Here's how the part is built. I have some questions about the finished solid (model axes, mm). Face numbers are marked on the shaded views. A direction names the side the tool comes from. Coordinates: 2 decimals unless noted, no trailing zeros. Write each loop counter-clockwise with the first axis right and the second up, starting at its lowest first coordinate (ties: lowest second). Pieces come first, ordered by that corner, then holes.
Item 1: I want a section at A-A (z = 7). Please give me the cut outline in (x, y), and give its area (3 significant figures).
Item 2: I'm going to push flat-ended pins straight in: P1, Ø12, axis at y = -29, z = 18.5, coming from the +X side; P2, Ø3, axis at x = -17, y = -10, coming from the +Z side; P3, Ø3, axis at x = 28, z = 13, coming from the +Y side; P4, Ø5, axis at x = -1.5, y = -7, coming from the -Z side. Where does each tip first touch, or does it pass through?
Item 3: I want a section at C-C (y = 18.5). Please give me the cut outline in (x, z).
Item 4: For the marked faces 5, 6, 7, 8 and 9, which set-ups out of +Z, -Z, +X, -X, +Y, -Y let a thin tool reach every point of the face, with its end or its side?
Item 5: I want a section at B-B (x = -13.5). Please give me the cut outline in (y, z).
Item 6: Please list where these lines run through material, in increasing order: line 1 (X direction, y = 6, z = 30.5); line 2 (X direction, y = 35.5, z = 6); line 3 (Y direction, x = -12.5, z = 32).
Item 7: I want a section at D-D (x = 24). Please give me the cut outline in (y, z), and give its area (3 significant figures).
Item 8: If we mould it in two halves opening along Y, with no side actions, what happens to the marked faces 1, 2, 3 and 4? For each: pulls with the +Y half, pulls with the -Y half, needs draft (parallel to the pull), parting line crosses it, or undercut.
from build123d import *

# Parameters (mm, degrees)
EXTRUDE_1_DEPTH     = 34
SKETCH_4_R          = 3.85
SKETCH_4_R_2        = 2.85
EXTRUDE_2_DEPTH     = 16.5
SKETCH_5_R          = 1.85
CUT_EXTRUDE_2_DEPTH = 35
SKETCH_6_R          = 3
CUT_EXTRUDE_3_DEPTH = 4
SKETCH_7_W          = 34
SKETCH_7_H          = 5
EXTRUDE_3_DEPTH     = 15
FILLET_2_R          = 2.5
FILLET_3_R          = 2.5
FILLET_4_R          = 2.5
SKETCH_8_W          = 5
SKETCH_8_H          = 34
EXTRUDE_4_DEPTH     = 15
SKETCH_9_W          = 5
SKETCH_9_H          = 34
EXTRUDE_5_DEPTH     = 15
FILLET_5_R          = 2.5


with BuildPart() as part:
    # 草圖1 → 填料-伸長1 (new body)
    with BuildSketch(Plane.XY):
        Polygon((0.59122025, -5.441901053), (39.56236342, -27.941901053), (36.06236342, -34.00407888), (-2.90877975, -11.50407888), (-41.87992292, -34.00407888), (-45.37992292, -27.941901053), (-6.40877975, -5.441901053), (-6.40877975, 39.558098947), (0.59122025, 39.558098947), align=None)
    extrude(amount=EXTRUDE_1_DEPTH)

    # 草圖4 → 填料-伸長2 (add)
    with BuildSketch(Plane.XY.offset(34)):
        with Locations((-2.90877975, -7.462626996)):
            Circle(SKETCH_4_R)
        with Locations((-2.90877975, -7.462626996)):
            Circle(SKETCH_4_R_2, mode=Mode.SUBTRACT)
    extrude(amount=EXTRUDE_2_DEPTH)

    # 草圖5 → 除料-伸長2 (cut, through all)
    with BuildSketch(Plane.XY.offset(34)):
        with Locations((-2.90877975, -7.462626996)):
            Circle(SKETCH_5_R)
    extrude(amount=-CUT_EXTRUDE_2_DEPTH, mode=Mode.SUBTRACT)

    # 草圖6 → 除料-伸長3 (cut)
    with BuildSketch(Plane(origin=(0, 0, 0), x_dir=(-1, 0, 0), z_dir=(0, 0, -1))):
        with Locations((2.90877975, -7.462626996)):
            Circle(SKETCH_6_R)
    extrude(amount=-CUT_EXTRUDE_3_DEPTH, mode=Mode.SUBTRACT)

    # 草圖7 → 填料-伸長3 (add)
    with BuildSketch(Plane.ZY.offset(6.40877975)):
        with Locations((17, 37.058098947)):
            Rectangle(SKETCH_7_W, SKETCH_7_H)
    extrude(amount=EXTRUDE_3_DEPTH)

    # 圓角2
    fillet_2_edges = [part.edges().sort_by_distance(p)[0] for p in [
        (-21.40877975, 39.558098947, 17),
    ]]
    fillet(fillet_2_edges, radius=FILLET_2_R)

    # 圓角3
    fillet_3_edges = [part.edges().sort_by_distance(p)[0] for p in [
        (0.59122025, 39.558098947, 17),
    ]]
    fillet(fillet_3_edges, radius=FILLET_3_R)

    # 圓角4
    fillet_4_edges = [part.edges().sort_by_distance(p)[0] for p in [
        (-6.40877975, 34.558098947, 17),
    ]]
    fillet(fillet_4_edges, radius=FILLET_4_R)

    # 草圖8 → 填料-伸長4 (add)
    with BuildSketch(Plane(origin=(4.254217341, -7.368520581, 0), x_dir=(0.866025404, 0.5, 0), z_dir=(0.5, -0.866025404, 0))):
        with Locations((-50.771116598, 17)):
            Rectangle(SKETCH_8_W, SKETCH_8_H)
    extrude(amount=EXTRUDE_4_DEPTH)

    # 草圖9 → 填料-伸長5 (add)
    with BuildSketch(Plane(origin=(-2.208607216, -3.825419912, 0), x_dir=(0.866025404, -0.5, 0), z_dir=(0.5, 0.866025404, 0))):
        with Locations((45.732962282, -17)):
            Rectangle(SKETCH_9_W, SKETCH_9_H)
    extrude(amount=EXTRUDE_5_DEPTH)

    # 圓角5
    fillet_5_edges = [part.edges().sort_by_distance(p)[0] for p in [
        (36.06236342, -34.00407888, 17),
        (-45.37992292, -27.941901053, 17),
        (-34.37992292, -46.994459937, 17),
        (47.06236342, -14.951519997, 17),
    ]]
    fillet(fillet_5_edges, radius=FILLET_5_R)


solid = part.part
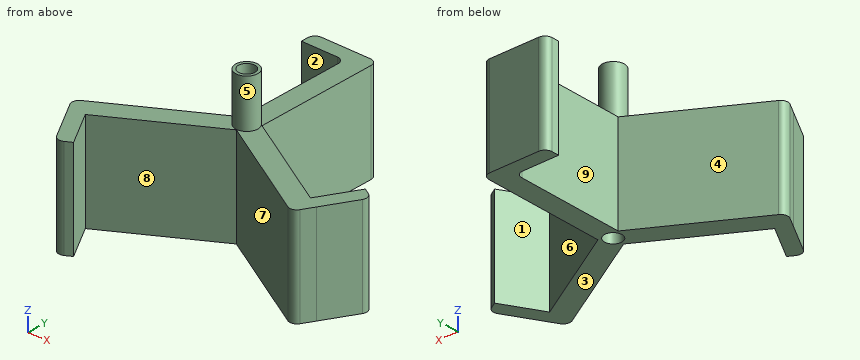
Answer:
1. outline: (-44.13, -30.11) - (-35.63, -44.83) arc R2.5 ccw to (-32.21, -45.74) - (-30.05, -44.49) - (-37.55, -31.5) - (-2.91, -11.5) - (33.9, -32.75) arc R2.5 ccw to (37.31, -31.84) - (45.81, -17.12) arc R2.5 ccw to (44.9, -13.7) - (42.73, -12.45) - (35.23, -25.44) - (0.59, -5.44) - (0.59, 37.06) arc R2.5 ccw to (-1.91, 39.56) - (-18.91, 39.56) arc R2.5 ccw to (-21.41, 37.06) - (-21.41, 34.56) - (-8.91, 34.56) arc R2.5 cw to (-6.41, 32.06) - (-6.41, -5.44) - (-43.21, -26.69) arc R2.5 ccw to start; hole circle Ø3.7 at (-2.91, -7.46)
1. area: 1,170 mm2
2. P1: stops at x = 42.42
2. P2: stops at z = 34
2. P3: stops at y = -20.4
2. P4: stops at z = 0
3. outline: (-6.41, 0) - (0.59, 0) - (0.59, 34) - (-6.41, 34) - close
4. face 5: +Z
4. face 6: +Z, -Z, +Y
4. face 7: +Z, -Z, -Y
4. face 8: +Z, -Z
4. face 9: +Z, -Z, -X
5. outline: (-17.62, 0) - (-9.54, 0) - (-9.54, 34) - (-17.62, 34) - close; (34.56, 0) - (39.56, 0) - (39.56, 34) - (34.56, 34) - close
6. line 1: x = -6.41 to 0.59
6. line 2: x = -21.41 to 0.59
6. line 3: y = -17.04 to -8.96, 34.56 to 39.56
7. outline: (-27.04, 0) - (-18.96, 0) - (-18.96, 34) - (-27.04, 34) - close
7. area: 275 mm2
8. face 1: pulls with the +Y half
8. face 2: undercut
8. face 3: needs draft
8. face 4: undercut
